Job drawing, mm, ordinate dimensions from the low corner. One solid piece. A direction names the side the tool comes from. Give positions to 0.01 mm unless a question says otherwise; leave off trailing zeros. Loops run counter-clockwise (first coordinate to the right, second up) from the corner with the lowest first, then second, coordinate; pieces in that order, holes last. Notation, with made-up numbers: M 35,-16 L 50,-16 A23 cw 50,-4 Z; hole C 42,58.25 d8. An arc over 180 degrees is marked long. Put each result on its own line as item: value.
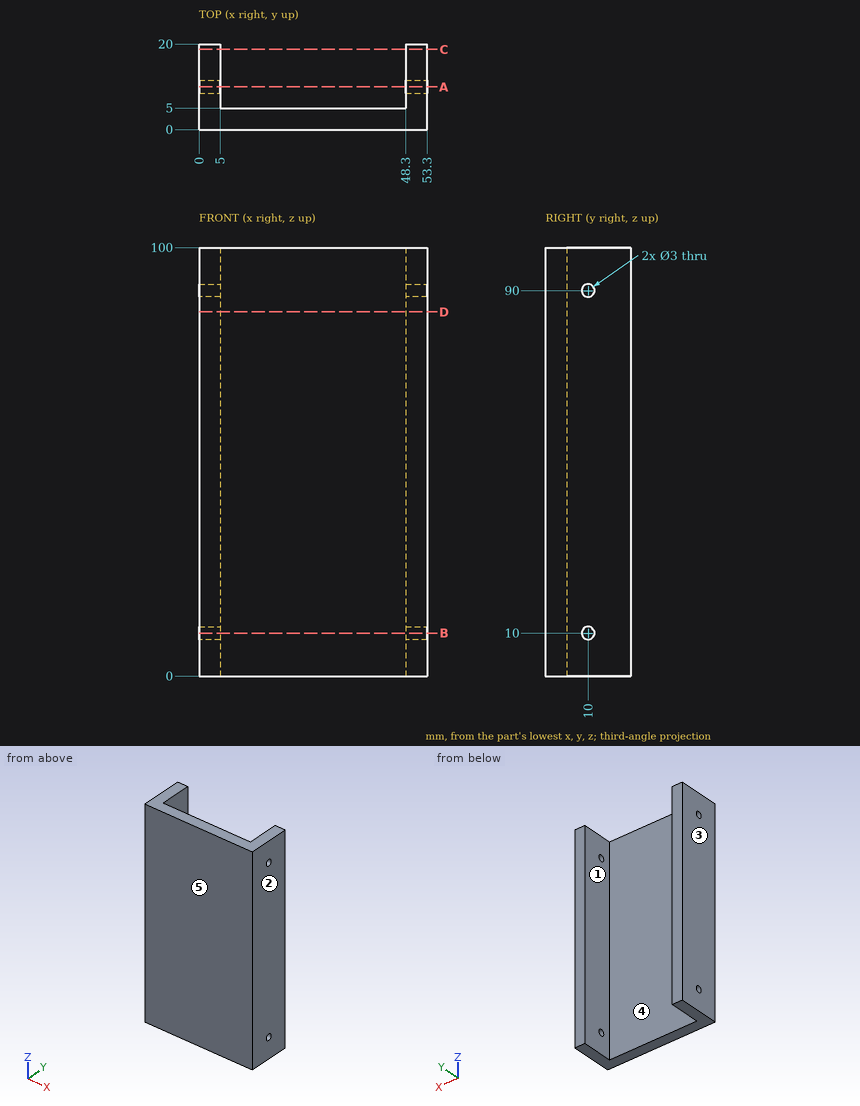
Q1. Drop flat-ended pins along their axis: pin 1 Ø2.5 at (y, z) = (10, 10) entering from +X; pin 2 Ø2 at (x, z) = (9, 81) entering from +Y. Give the stop position or say it passes through.
Here are the results:
pin 1: through
pin 2: y = 5
Q2. Probe line 1 (X direction, y = 7, z = 82); line 2 (Y direction, x = 50.8, z = 90); line 3 (Y direction, x = 21.5, z = 26). List the from-to ranges inside material, lowest first. Write a range as from..to.
Here are the results:
line 1: 0..5, 48.3..53.3
line 2: 0..8.5, 11.5..20
line 3: 0..5
Q3. Slice it at D-D (z = 85). List the corners of the cut face in (x, y).
Here are the results:
outline: M 0,0 L 53.3,0 L 53.3,20 L 48.3,20 L 48.3,5 L 5,5 L 5,20 L 0,20 Z
Q4. Slice it at C-C (y = 18.75). List the corners of the cut face in (x, z), and give its area (3 significant figures).
Here are the results:
outline: M 0,0 L 5,0 L 5,100 L 0,100 Z; M 48.3,0 L 53.3,0 L 53.3,100 L 48.3,100 Z
area: 1,000 mm²
Q5. Slice it at B-B (z = 10). List the corners of the cut face in (x, y), and give its area (4 significant figures).
Here are the results:
outline: M 0,0 L 53.3,0 L 53.3,8.5 L 48.3,8.5 L 48.3,5 L 5,5 L 5,8.5 L 0,8.5 Z; M 0,11.5 L 5,11.5 L 5,20 L 0,20 Z; M 48.3,11.5 L 53.3,11.5 L 53.3,20 L 48.3,20 Z
area: 386.5 mm²
Q6. Mould opens along X. For the marked faces 1, 2 and 3 say: pulls with the +X half, pulls with the -X half, needs draft (parallel to the pull), parting line crosses it, or undercut.
Here are the results:
face 1: undercut
face 2: pulls with the +X half
face 3: pulls with the -X half
Q7. Tool access for the marked faces 4 and 5: list every direction of +Z, -Z, +X, -X, +Y, -Y with a clear straight run to the whole face (end or side of a thin tool).
Here are the results:
face 4: +Z, -Z, +Y
face 5: +Z, -Z, +X, -X, -Y
Q8. Slice it at A-A (y = 10). List the corners of the cut face in (x, z), and give its area (3 significant figures).
Here are the results:
outline: M 0,0 L 5,0 L 5,8.5 L 0,8.5 Z; M 0,11.5 L 5,11.5 L 5,88.5 L 0,88.5 Z; M 0,91.5 L 5,91.5 L 5,100 L 0,100 Z; M 48.3,0 L 53.3,0 L 53.3,8.5 L 48.3,8.5 Z; M 48.3,11.5 L 53.3,11.5 L 53.3,88.5 L 48.3,88.5 Z; M 48.3,91.5 L 53.3,91.5 L 53.3,100 L 48.3,100 Z
area: 940 mm²
